For this review, take the finished solid that the model builds, in its own axes (mm). Face numbers are marked on the shaded views. A direction names the side the tool comes from. Coordinates: 2 decimals unless noted, no trailing zeros. Loops run counter-clockwise (first coordinate to the right, second up) from the corner with the lowest first, then second, coordinate; pieces in that order, holes last. Notation, with made-up numbers: (74, 27.5) -> (124, 27.5) arc R23 cw to (124, 63.5) -> close; hole circle Ø11 at (-38, 23). An arc over 180 degrees is marked (long way). Use a Markdown table: item, result.
from build123d import *

# Parameters (mm, degrees)
F0_W     = 360
F0_H     = 360
F1_DEPTH = 30
F2_W     = 360
F2_H     = 360
F2_W_2   = 80
F2_H_2   = 100
F3_DEPTH = 33


with BuildPart() as f1:
    # F0 (on Top) → F1 (new body)
    with BuildSketch(Plane.XY):
        Rectangle(F0_W, F0_H)
    extrude(amount=F1_DEPTH)

    # F2 (on face) → F3 (join)
    with BuildSketch(Plane(origin=(0, 0, 0), x_dir=(1, 0, 0), z_dir=(0, 0, -1))):
        Rectangle(F2_W, F2_H)
        with Locations((-100, 0)):
            Rectangle(F2_W_2, F2_H_2, mode=Mode.SUBTRACT)
        with Locations((100, 0)):
            Rectangle(F2_W_2, F2_H_2, mode=Mode.SUBTRACT)
    extrude(amount=F3_DEPTH)


solid = f1.part
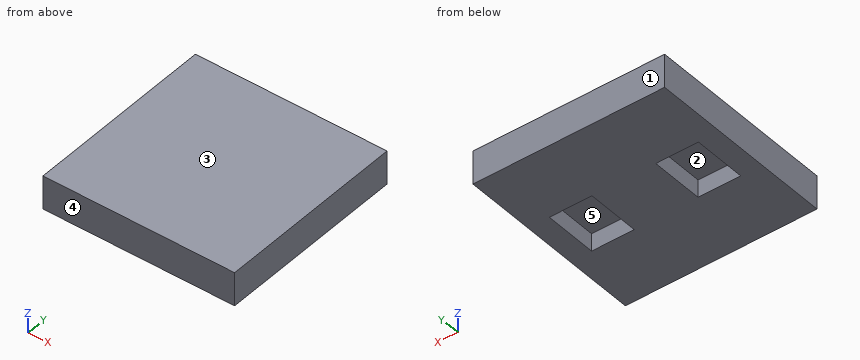
(1) Take a section at C-C on x = 91.5. Write out the cut boundary in (y, z), plus the area to 3 significant figures.
Found:
| item | result |
|---|---|
| outline | (-180, -33) -> (-50, -33) -> (-50, 0) -> (50, 0) -> (50, -33) -> (180, -33) -> (180, 30) -> (-180, 30) -> close |
| area | 19,400 mm^2 |
(2) Take a section at A-A on z = -26.5. Write out the cut boundary in (x, y), plus the area to 3 significant figures.
Found:
| item | result |
|---|---|
| outline | (-180, -180) -> (180, -180) -> (180, 180) -> (-180, 180) -> close; hole (-140, -50) -> (-60, -50) -> (-60, 50) -> (-140, 50) -> close; hole (60, -50) -> (140, -50) -> (140, 50) -> (60, 50) -> close |
| area | 114,000 mm^2 |
(3) Take a section at B-B on y = 29.5. Write out the cut boundary in (x, z).
Found:
| item | result |
|---|---|
| outline | (-180, -33) -> (-140, -33) -> (-140, 0) -> (-60, 0) -> (-60, -33) -> (60, -33) -> (60, 0) -> (140, 0) -> (140, -33) -> (180, -33) -> (180, 30) -> (-180, 30) -> close |
(4) For line 1 along X through (y, z) = (30, -22); line 2 along Z through (x, y) = (94, 25.5); line 3 along Y through (x, z) = (139.5, -18), list the stretches that pass through material, from the lowest coordinate up.
Found:
| item | result |
|---|---|
| line 1 | x = -180 to -140, -60 to 60, 140 to 180 |
| line 2 | z = 0 to 30 |
| line 3 | y = -180 to -50, 50 to 180 |
(5) Mouldability with a two-part tool opening along Y and no side actions: class the marked faces 3, 4 and 5 as pulls with the +Y half, pulls with the -Y half, needs draft (parallel to the pull), parting line crosses it, or undercut.
Found:
| item | result |
|---|---|
| face 3 | needs draft |
| face 4 | pulls with the -Y half |
| face 5 | undercut |
(6) For the marked faces 1 and 2, list the 3-axis set-ups (+Z, -Z, +X, -X, +Y, -Y) from which the entire face can be reached by the end or side of a thin tool; tool diameter is ignored.
Found:
| item | result |
|---|---|
| face 1 | +Z, -Z, +X, -X, +Y |
| face 2 | -Z |
